from build123d import *

# Parameters (mm, degrees)
SKETCH1_W           = 120
SKETCH1_H           = 80
SKETCH1_W_2         = 102
SKETCH1_H_2         = 62
BOSS_EXTRUDE1_DEPTH = 60
SKETCH2_W           = 120
SKETCH2_H           = 80
BOSS_EXTRUDE2_DEPTH = 5
SKETCH5_R           = 2.6
CUT_EXTRUDE1_DEPTH  = 141
SKETCH6_R           = 5
CUT_EXTRUDE2_DEPTH  = 94.808315196
SKETCH7_W           = 26.53085
SKETCH7_H           = 10
BOSS_EXTRUDE3_DEPTH = 15
SKETCH8_W           = 4
SKETCH8_H           = 6.5
SKETCH8_R           = 1.5
CUT_EXTRUDE3_DEPTH  = 10


with BuildPart() as part:
    # Sketch1 → Boss-Extrude1 (new body)
    with BuildSketch(Plane(origin=(0, 0, 0), x_dir=(1, 0, 0), z_dir=(0, 1, 0))):
        Rectangle(SKETCH1_W, SKETCH1_H)
        Rectangle(SKETCH1_W_2, SKETCH1_H_2, mode=Mode.SUBTRACT)
    extrude(amount=BOSS_EXTRUDE1_DEPTH)

    # Sketch2 → Boss-Extrude2 (add)
    with BuildSketch(Plane.XZ):
        Rectangle(SKETCH2_W, SKETCH2_H)
    extrude(amount=BOSS_EXTRUDE2_DEPTH)

    # Sketch5 → Cut-Extrude1 (cut, through all)
    with BuildSketch(Plane.ZY.offset(60)):
        with Locations((-20, 50.5)):
            Circle(SKETCH5_R)
        with Locations((20, 50.25689587)):
            Circle(SKETCH5_R)
        with Locations((-20, 7)):
            Circle(SKETCH5_R)
        with Locations((19.471268046, 6.760109293)):
            Circle(SKETCH5_R)
    extrude(amount=-CUT_EXTRUDE1_DEPTH, mode=Mode.SUBTRACT)

    # Sketch6 → Cut-Extrude2 (cut, through all)
    with BuildSketch(Plane(origin=(0, 0, 0), x_dir=(1, 0, 0), z_dir=(0, 1, 0))):
        with Locations(Location((0, 0, 0), (0, 0, 270))):
            Circle(SKETCH6_R)
    extrude(amount=-CUT_EXTRUDE2_DEPTH, mode=Mode.SUBTRACT)

    # Sketch7 → Boss-Extrude3 (add)
    with BuildSketch(Plane.XZ.offset(5)):
        with Locations((0, -15)):
            Rectangle(SKETCH7_W, SKETCH7_H)
    extrude(amount=BOSS_EXTRUDE3_DEPTH)

    # Sketch8 → Cut-Extrude3 (cut)
    with BuildSketch(Plane.XZ.offset(20)):
        with Locations((0, -13.25)):
            Rectangle(SKETCH8_W, SKETCH8_H)
        with Locations(Location((-5.000005, -14.5, 0), (0, 0, 270))):
            Circle(SKETCH8_R)
        with Locations(Location((5.000005, -14.5, 0), (0, 0, 270))):
            Circle(SKETCH8_R)
    extrude(amount=-CUT_EXTRUDE3_DEPTH, mode=Mode.SUBTRACT)


solid = part.part
Design review of the part built by this model. Coordinates are the model's own, in mm. A direction names the side the tool comes from. Round coordinates to 2 decimals unless told otherwise and drop trailing zeros. Write each loop counter-clockwise with the first axis right and the second up, starting at its lowest first coordinate (ties: lowest second). Pieces come first, ordered by that corner, then holes. Notation, with made-up numbers: (15.25, 16.25) - (72.25, 16.25) arc R28 cw to (72.25, 48.25) - close; hole circle Ø10 at (7, 69). An arc over 180 degrees is marked (long way). Use a Markdown table: item, result. Add a question column.
1. For faces 1 (the face through (0, -12, -20)), 2 (the face through (-3, -12, -10)), 3 (the face through (2, -15, -13)), 4 (the face through (-1, 30, -31)), 5 (the face through (4.1, -15.1, -13.3)), list the 3-axis set-ups (+Z, -Z, +X, -X, +Y, -Y) from which the entire face can be reached by the end or side of a thin tool; tool diameter is ignored.
2. We need section B-B (x = 0). State the section outline as (y, z) points, then the cut area to 4 significant figures.
3. Wall thickness on probe 1 along Y at (x, z) = (-55.5, -20); probe 2 along Z at (x, y) = (-45.5, 9); probe 3 along X at (y, z) = (42, -25): over which ranges is each line inside the solid? List them lowest first.
4. We need section D-D (z = 12). State the section outline as (x, y) points.
5. Mouldability with a two-part tool opening along X and no side actions: class faces 6 (the face through (-1, -5, 9)), 7 (the face through (0, -10, -13)), 8 (the face through (-13.265, -12, -15)) as +X half, -X half, draft (parallel to the pull), parting line (faces both ways), or undercut.
6. We need section C-C (y = 43.5). State the section outline as (x, z) points, then the cut area to 3 significant figures.
7. We need section A-A (z = 0). State the section outline as (x, y) points, then the cut area to 3 significant figures.
8. Clearance check with flat-ended pins moving along their axes: pin 1 (11.5 mm diameter, centred on x = 0, z = 0, fed in from +Y); pin 2 (1.5 mm diameter, centred on x = 5.5, z = -14.5, fed in from -Y); pin 3 (3 mm diameter, centred on x = 1, y = -14, fed in from +Z). State where each tip first meets the part, or that it passes through.
Output:
| question | item | result |
|---|---|---|
| 1 | face 1 | -Z, +X, -X, -Y |
| 1 | face 2 | +Z, +X, -X, -Y |
| 1 | face 3 | +Z, -Y |
| 1 | face 4 | +Y |
| 1 | face 5 | -Y |
| 2 | outline | (-20, -20) - (-5, -20) - (-5, -40) - (60, -40) - (60, -31) - (0, -31) - (0, -5) - (-5, -5) - (-5, -10) - (-10, -10) - (-10, -16.5) - (-20, -16.5) - close; (-5, 5) - (0, 5) - (0, 31) - (60, 31) - (60, 40) - (-5, 40) - close |
| 2 | area | 1,515 mm2 |
| 3 | probe 1 | y = -5 to 4.4, 9.6 to 47.9, 53.1 to 60 |
| 3 | probe 2 | z = -40 to -31, 31 to 40 |
| 3 | probe 3 | x = -60 to -51, 51 to 60 |
| 4 | outline | (-60, -5) - (60, -5) - (60, 60) - (51, 60) - (51, 0) - (-51, 0) - (-51, 60) - (-60, 60) - close |
| 5 | face 6 | draft |
| 5 | face 7 | undercut |
| 5 | face 8 | -X half |
| 6 | outline | (-60, -40) - (60, -40) - (60, 40) - (-60, 40) - close; hole (-51, -31) - (51, -31) - (51, 31) - (-51, 31) - close |
| 6 | area | 3,280 mm2 |
| 7 | outline | (-60, -5) - (-5, -5) - (-5, 0) - (-51, 0) - (-51, 60) - (-60, 60) - close; (5, -5) - (60, -5) - (60, 60) - (51, 60) - (51, 0) - (5, 0) - close |
| 7 | area | 1,630 mm2 |
| 8 | pin 1 | stops at y = 0 |
| 8 | pin 2 | stops at y = -10 |
| 8 | pin 3 | stops at z = -10 |
